Autodesk Inventor part; units mm, degrees
ref_plane "YZ Plane" through (0, 0, 0) normal (1, 0, 0) x (0, 1, 0)
ref_plane "XZ Plane" through (0, 0, 0) normal (0, 1, 0) x (-1, 0, 0)
ref_plane "XY Plane" through (0, 0, 0) normal (0, 0, 1) x (1, 0, 0)
sketch "Sketch1" plane through (0, 0, 0) normal (0, 1, 0) x (-1, 0, 0)
  line L0 (35, 35) -> (35, 3)
  line L1 (9, 3) -> (35, 3) construction
  line L2 (0, 3) -> (9, 3) construction
  line L3 (35, 3) -> (50, 3)
  line L4 (0, -35) -> (0, 35)
  line L5 (0, -35) -> (50, -35)
  line L6 (0, 35) -> (35, 35)
  line L7 (50, -35) -> (50, 3)
  line L8 (30.7, 28.05) -> (35, 28.05) construction
  line L9 (30.7, 28.05) -> (30.7, 9.95) construction
  line L10 (30.7, 9.95) -> (30.7, 3) construction
  circle A0 centre (30.7, 9.95) radius 1.25
  circle A1 centre (30.7, 28.05) radius 1.25
  circle A2 centre (44, -3) radius 1.25
  arc A3 (0, -31.25) -> (0, -28.75) centre (0, -30) ccw
  arc A4 (0, 6.45) -> (0, 8.95) centre (0, 7.7) ccw
  arc A5 (0, 28.05) -> (0, 30.55) centre (0, 29.3) ccw
  line L11 (0, 29.3) -> (30.7, 29.3) construction
  line L12 (50, -35) -> (50, -65)
  line L13 (50, -65) -> (0, -65)
  line L14 (0, -35) -> (0, -65)
  circle A6 centre (44, -41) radius 1.25
  circle A7 centre (18, -41) radius 1.25
  circle A8 centre (18, -51) radius 1.25
  point P0 (0, 0)
  point P1 (-50, 0)
  point P2 (0, 0)
  dimension "d26" = 2.5
  dimension "d6" = 32
  dimension "d9" = 26
  dimension "d10" = 9
  dimension "d11" = 50
  dimension "d12" = 70
  dimension "d14" = 4.3
  dimension "d15" = 18.1
  dimension "d20" = 6.95
  dimension "d25" = 2.5
  dimension "d32" = 2.5
  dimension "d33" = 2.5
  dimension "d35" = 2.5
  dimension "d36" = 30
  dimension "d37" = 6
  dimension "d38" = 6
  dimension "d39" = 32
  dimension "d40" = 10
  dimension "d41" = 2.5
  dimension "d42" = 2.5
  dimension "d43" = 2.5
  dimension "d55" = 6
  dimension "d56" = 6
  dimension "d57" = 2.5
  dimension "d58" = 5
  dimension "d59" = 2.25
extrude "Extrusion1" add sketch "Sketch1" along normal blind 3 contours L0 L3 L7 L5 L4 A3 A4 A5 L6 | A5 L4 | L12 L13 L14 L5 | A4 L4 | L4 A3 | A0 | A1 | A2
extrude "Extrusion4" cut sketch "Sketch1" along normal through all contours A5 L4 | A4 L4 | L4 A3 | A0 | A1 | A2
mirror "Mirror1" about plane through (0, 0, 0) normal (1, 0, 0) of "Extrusion1", "Extrusion4"
sketch "Sketch4" plane through (-50, 0, -65) normal (-1, 0, 0) x (0, 0, 1)
  line L0 (0, 3) -> (68, 3)
  line L1 (0, 3) -> (3, 3)
  line L2 (0, 0) -> (68, 0)
  line L3 (3, 3) -> (0, 0)
  line L4 (0, 0) -> (0, 3)
  line L5 (0, 0) -> (0, 3)
  point P0 (65, 0)
  dimension "d44" = 3
extrude "Extrusion5" cut sketch "Sketch4" against normal through all
sketch "Sketch5" plane through (0, 3, 0) normal (0, 1, 0) x (1, 0, 0)
  circle A0 centre (-40, 49) radius 6
  line L0 (-50, 62) -> (-50, -3)
  line L1 (50, 62) -> (-50, 62)
  point P0 (0, 0)
  dimension "d50" = 10
  dimension "d51" = 13
  dimension "d52" = 12
extrude "Extrusion6" cut sketch "Sketch5" against normal through all
mirror "Mirror2" about plane through (0, 0, 0) normal (1, 0, 0) of "Extrusion6"
properties part number "Podstawa_All_in_One_3mm"
Geometry check sheet. Reference: the model listing, model coordinates, mm. A direction names the side the tool comes from. Coordinates: 2 decimals unless noted, no trailing zeros. Loops run counter-clockwise (first coordinate to the right, second up) from the corner with the lowest first, then second, coordinate; pieces in that order, holes last.
Item 1: Access from +Z, -Z, +X, -X, +Y, -Y to the whole of each face (thin tool, end or side, straight path). Record for faces 1 (the face through (-35, 1, 19)), 2 (the face through (1, 3, -13)).
Item 2: Thickness scan on line 1 (X direction, y = 1.5, z = -53.5); line 2 (X direction, y = 0.4, z = 9.5); line 3 (Z direction, x = 0, y = 0.8). Record the ranges inside material, lowest first.
Item 3: Release check for a two-part mould opening along X. For faces 3 (the face through (35, 1, 19)), 4 (the face through (29.45, 1.48, 28.1)), 5 (the face through (-42, 1, 3)) record: released by +X, released by -X, zero draft, split by the parting line, or undercut.
Item 4: Sectioned sample at D-D, the plane y = 0.65. Count the separate pieces of the cut face and the enclosed holes in it, then the cut area to 3 significant figures.
Item 5: Sectioned sample at B-B, the plane x = 0. Record the boundary of the cut face in (y, z), then the cut area to 3 significant figures.
Item 6: Sectioned sample at A-A, the plane z = -3. Record the boundary of the cut face in (x, y).
Item 7: Sectioned sample at C-C, the plane z = -41. Record the boundary of the cut face in (x, y).
Item 8: Go/stop test with flat-tipped pins: pin 1 Ø2 at (x, z) = (-18, -51) entering from +Y; pin 2 Ø0.9 at (x, y) = (44.5, 1.5) entering from +Z. Record where each tip stops, or that it passes through.
Check result:
1. face 1: +Z, -X, +Y, -Y
1. face 2: +Z, -Z, +X, -X, +Y
2. line 1: x = -50 to -43.97, -36.03 to 36.03, 43.97 to 50
2. line 2: x = -35 to -31.87, -29.53 to 29.53, 31.87 to 35
2. line 3: z = -64.2 to -31.25, -28.75 to 6.45, 8.95 to 28.05, 30.55 to 35
3. face 3: released by +X
3. face 4: undercut
3. face 5: zero draft
4. separate pieces: 1
4. enclosed holes: 17
4. area: 8,680 mm2
5. outline: (0, -65) - (3, -62) - (3, -31.25) - (0, -31.25) - close; (0, -28.75) - (3, -28.75) - (3, 6.45) - (0, 6.45) - close; (0, 8.95) - (3, 8.95) - (3, 28.05) - (0, 28.05) - close; (0, 30.55) - (3, 30.55) - (3, 35) - (0, 35) - close
5. area: 273 mm2
6. outline: (-50, 0) - (-45.25, 0) - (-45.25, 3) - (-50, 3) - close; (-42.75, 0) - (42.75, 0) - (42.75, 3) - (-42.75, 3) - close; (45.25, 0) - (50, 0) - (50, 3) - (45.25, 3) - close
7. outline: (-50, 0) - (-45.25, 0) - (-45.25, 3) - (-50, 3) - close; (-42.75, 0) - (-19.25, 0) - (-19.25, 3) - (-42.75, 3) - close; (-16.75, 0) - (16.75, 0) - (16.75, 3) - (-16.75, 3) - close; (19.25, 0) - (42.75, 0) - (42.75, 3) - (19.25, 3) - close; (45.25, 0) - (50, 0) - (50, 3) - (45.25, 3) - close
8. pin 1: passes through
8. pin 2: stops at z = 3
